Could you check a few things on this drawing? It's one solid part, dimensions in mm from its lowest x, y, z. Give positions to 0.01 mm unless a question says otherwise; leave off trailing zeros. Loops run counter-clockwise (first coordinate to the right, second up) from the corner with the lowest first, then second, coordinate; pieces in that order, holes last. Notation, with made-up numbers: M 67.25,20.5 L 74.25,20.5 A15 cw 74.25,43.5 Z; hole C 45,-36 d9. An arc over 180 degrees is marked long. Return JSON: item names as keys, results as strings. Group by question number.
1. If we section it at B-B (x = 37): Write out the boundary of the cut face in (y, z).
2. Please list where these lines run through material, in increasing order: line 1 (Y direction, x = 68, z = 0.9); line 2 (Y direction, x = 5.5, z = 0.9); line 3 (X direction, y = 15, z = 1.35).
3. If we section it at D-D (y = 10.5): Write out the boundary of the cut face in (x, z).
4. If we section it at C-C (z = 1.1): Write out the boundary of the cut face in (x, y).
5. If we section it at A-A (y = 17.5): Write out the boundary of the cut face in (x, z), plus the area to 4 significant figures.
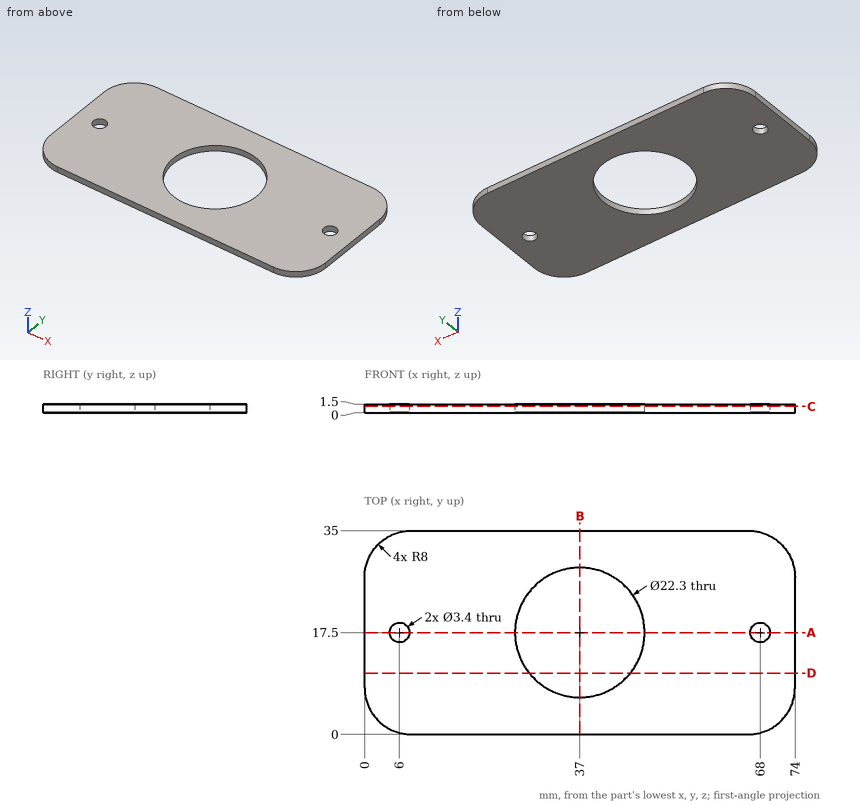
Answer:
{
 "1": {"outline": "M 0,0 L 6.35,0 L 6.35,1.5 L 0,1.5 Z; M 28.65,0 L 35,0 L 35,1.5 L 28.65,1.5 Z"},
 "2": {"line 1": "y = 0.25 to 15.8, 19.2 to 34.75", "line 2": "y = 0.4 to 15.88, 19.12 to 34.6", "line 3": "x = 0 to 26.13, 47.87 to 74"},
 "3": {"outline": "M 0,0 L 28.32,0 L 28.32,1.5 L 0,1.5 Z; M 45.68,0 L 74,0 L 74,1.5 L 45.68,1.5 Z"},
 "4": {"outline": "M 0,8 A8 ccw 8,0 L 66,0 A8 ccw 74,8 L 74,27 A8 ccw 66,35 L 8,35 A8 ccw 0,27 Z; hole C 6,17.5 d3.4; hole C 37,17.5 d22.3; hole C 68,17.5 d3.4"},
 "5": {"outline": "M 0,0 L 4.3,0 L 4.3,1.5 L 0,1.5 Z; M 7.7,0 L 25.85,0 L 25.85,1.5 L 7.7,1.5 Z; M 48.15,0 L 66.3,0 L 66.3,1.5 L 48.15,1.5 Z; M 69.7,0 L 74,0 L 74,1.5 L 69.7,1.5 Z", "area": "67.35 mm²"}
}
